Geometry: final body of the model. Coordinates: model frame, mm. Face numbers are marked on the shaded views. A direction names the side the tool comes from. Coordinates: 2 decimals unless noted, no trailing zeros. Write each loop counter-clockwise with the first axis right and the second up, starting at its lowest first coordinate (ties: lowest second). Pieces come first, ordered by that corner, then holes.
from build123d import *

# Parameters (mm, degrees)
PAD002_DEPTH       = 10
SKETCH027_R        = 3.6
POCKET001_DEPTH    = 5
POCKET004_DEPTH    = 7
POLARPATTERN_COUNT = 6
SKETCH032_R        = 21.5
POCKET005_DEPTH    = 7
POCKET006_DEPTH    = 142.501
SKETCH034_W        = 5
SKETCH034_H        = 8.75
POCKET007_DEPTH    = 2
SKETCH029_R        = 1.4
POCKET010_DEPTH    = 142.501
SKETCH077_R        = 4.05
POCKET021_DEPTH    = 3
SKETCH080_R        = 5.05
SKETCH080_R_2      = 4.05
PAD026_DEPTH       = 2


with BuildPart() as part:
    # Sketch026 → Pad002 (new body)
    with BuildSketch(Plane.XY):
        with BuildLine():
            Line((-32.691742, 67.5), (-67.25, 67.5))
            Line((-67.25, 67.5), (-67.25, 87.5))
            Line((-67.25, 87.5), (67.25, 87.5))
            Line((67.25, 87.5), (67.25, 67.5))
            Line((67.25, 67.5), (32.691742, 67.5))
            ThreePointArc((61.712741, -42.620858), (72.523806, 19.112758), (32.691742, 67.5))
            ThreePointArc((42.620858, -61.712741), (61.712741, -61.712741), (61.712741, -42.620858))
            ThreePointArc((20, -72.284161), (31.753452, -67.946437), (42.620858, -61.712741))
            Line((20, -71.284161), (20, -72.284161))
            Line((-20, -71.284161), (20, -71.284161))
            Line((-20, -72.284161), (-20, -71.284161))
            ThreePointArc((-32.691742, 67.5), (-74.692756, -6.78175), (-20, -72.284161))
        make_face()
    extrude(amount=PAD002_DEPTH)

    # Sketch027 (on DatumPlane) → Pocket001 (cut)
    with BuildSketch(Plane.YZ.offset(67.5)):
        Polygon((74.25, 10), (87.5, 10), (87.5, 0), (82.25, 0), (74.25, 0), align=None)
        with Locations((82.25, 5.25)):
            Circle(SKETCH027_R, mode=Mode.SUBTRACT)
    pocket001 = extrude(amount=-POCKET001_DEPTH, mode=Mode.SUBTRACT)

    # Mirrored002: Pocket001 across YZ
    add(pocket001.mirror(Plane.YZ), mode=Mode.SUBTRACT)

    # Sketch030 → Groove (revolve, cut)
    with BuildSketch(Plane.XZ):
        with BuildLine():
            ThreePointArc((70, 0), (68, 4), (66, 0))
            Line((66, 0), (70, 0))
        make_face()
    revolve(axis=Axis((0, 0, 0), (0, 0, 1)), mode=Mode.SUBTRACT)

    # Sketch031 → Pocket004 (cut)
    with BuildSketch(Plane.XY):
        with BuildLine():
            ThreePointArc((49.255383, 39.279858), (27.334676, 56.761039), (0, 63))
            Line((0, 22.5), (0, 63))
            ThreePointArc((17.591208, 14.028521), (9.762384, 20.2718), (0, 22.5))
            Line((17.591208, 14.028521), (49.255383, 39.279858))
        make_face()
    pocket004 = extrude(amount=POCKET004_DEPTH, mode=Mode.SUBTRACT)

    # PolarPattern: Pocket004 ×6 about axis
    polarpattern_axis = Axis((0, 0, 0), (0, 0, 1))
    for i in range(1, POLARPATTERN_COUNT):
        add(pocket004.rotate(polarpattern_axis, i * 360 / POLARPATTERN_COUNT), mode=Mode.SUBTRACT)

    # Sketch032 → Pocket005 (cut)
    with BuildSketch(Plane.XY):
        Circle(SKETCH032_R)
    extrude(amount=POCKET005_DEPTH, mode=Mode.SUBTRACT)

    # Sketch033 (on DatumPlane) → Pocket006 (cut, through all)
    with BuildSketch(Plane.YZ.offset(67.5)):
        with BuildLine():
            Line((82.25, 0), (87.5, 0))
            Line((87.5, 0), (87.5, 5.25))
            ThreePointArc((82.25, 0), (85.962311, 1.537689), (87.5, 5.25))
        make_face()
    extrude(amount=-POCKET006_DEPTH, mode=Mode.SUBTRACT)

    # Sketch034 → Pocket007 (cut)
    with BuildSketch(Plane.XY):
        with Locations((64.75, 71.875)):
            Rectangle(SKETCH034_W, SKETCH034_H)
    pocket007 = extrude(amount=POCKET007_DEPTH, mode=Mode.SUBTRACT)

    # Mirrored003: Pocket007 across YZ
    add(pocket007.mirror(Plane.YZ), mode=Mode.SUBTRACT)

    # Sketch029 (on DatumPlane) → Pocket010 (cut, through all)
    with BuildSketch(Plane.YZ.offset(67.5)):
        with Locations((82.25, 5)):
            Circle(SKETCH029_R)
    extrude(amount=-POCKET010_DEPTH, mode=Mode.SUBTRACT)

    # Sketch077 (on DatumPlane) → Pocket021 (cut)
    with BuildSketch(Plane.XY.offset(-2)):
        with Locations((54.270445, -54.270445)):
            Circle(SKETCH077_R)
    extrude(amount=POCKET021_DEPTH, mode=Mode.SUBTRACT)

    # Sketch080 → Pad026 (join)
    with BuildSketch(Plane.XY):
        with Locations((54.270445, -54.270445)):
            Circle(SKETCH080_R)
        with Locations((54.270445, -54.270445)):
            Circle(SKETCH080_R_2, mode=Mode.SUBTRACT)
    extrude(amount=-PAD026_DEPTH)


with BuildPart() as part_1:
    # Body placement: moved
    add(part.part.moved(Location((0, 0, 10.5))))


solid = part_1.part
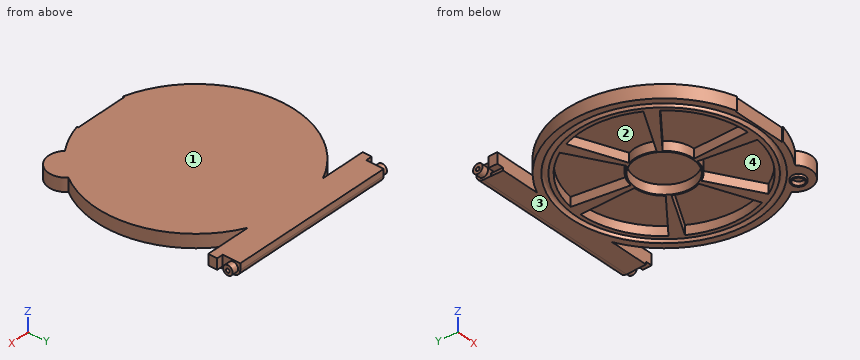
Item 1: Section B-B, the plane x = -36.5. State how many separate pieces and enclosed holes the cut face has, plus the area to 3 significant figures.
Derived:
separate pieces: 2
enclosed holes: 1
area: 843 mm2
Item 2: Pull-direction query (X, two-part tool) for the marked faces 3 and 4; classes: released by +X, released by -X, zero draft, split by the parting line, or undercut.
Derived:
face 3: zero draft
face 4: undercut
Item 3: Section A-A, the plane y = 0. Output: boundary loops of the cut face in (x, z).
Derived:
outline: (-75, 10.5) - (-70, 10.5) arc R2.5 cw (long way) to (-66, 10.5) - (-63, 10.5) - (-63, 17.5) - (-22.5, 17.5) - (-22.5, 10.5) - (-21.5, 10.5) - (-21.5, 17.5) - (21.5, 17.5) - (21.5, 10.5) - (22.5, 10.5) - (22.5, 17.5) - (63, 17.5) - (63, 10.5) - (66, 10.5) arc R2.5 cw (long way) to (70, 10.5) - (75, 10.5) - (75, 20.5) - (-75, 20.5) - close
Item 4: Pin query (flat end, axial travel): pin 1 (1.5 mm diameter, centred on x = -4, y = 67, fed in from -Z); pin 2 (1.5 mm diameter, centred on x = 4.5, z = 13.5, fed in from +Y); pin 3 (5 mm diameter, centred on y = 11.5, z = 19, fed in from -X). Return the tip coordinate at first contact, or that it passes through.
Derived:
pin 1: stops at z = 13.89
pin 2: stops at y = 87.28
pin 3: stops at x = -74.46
Item 5: Set-up query: the marked faces 1 and 2. Return all of +Z, -Z, +X, -X, +Y, -Y with unobstructed straight access to the full face (end or side cutting, diameter ignored); none if empty.
Derived:
face 1: +Z, +X, -X, +Y, -Y
face 2: -Z
Item 6: Material intervals for probe 1 along X at (y, z) = (32, 13); probe 2 along Y at (x, z) = (30, 17); probe 3 along Y at (x, z) = (25.5, 16), sorted ascending.
Derived:
probe 1: x = -67.83 to -62.58, -57.39 to -54.27, -4.82 to 0, 40.13 to 57.39, 62.58 to 67.83
probe 2: y = -68.74 to -55.4, -17.32 to -11.77, 17.32 to 23.92, 55.4 to 87.5
probe 3: y = -70.53 to -57.61, -14.72 to -10.01, 14.72 to 20.34, 57.61 to 80.94, 83.56 to 87.5
